```python
from build123d import *

# Parameters (mm, degrees)
F0_W     = 67
F0_H     = 88
F1_DEPTH = 3
F2_R     = 3.9
F3_DEPTH = 3.81
F5_D     = 3.5


with BuildPart() as f1:
    # F0 (on Top) → F1 (new body)
    with BuildSketch(Plane.XY):
        Rectangle(F0_W, F0_H)
    extrude(amount=F1_DEPTH)

    # F2 (on face) → F3 (join)
    with BuildSketch(Plane.XY.offset(3)):
        with Locations((-29.5, 40)):
            Circle(F2_R)
        with Locations((29.5, 40)):
            Circle(F2_R)
        with Locations((-29.5, -40)):
            Circle(F2_R)
        with Locations((29.5, -40)):
            Circle(F2_R)
    extrude(amount=F3_DEPTH)

    # F5 (through all)
    with Locations(Plane(origin=(0, 0, 0), x_dir=(1, 0, 0), z_dir=(0, 0, -1))):
        with Locations((29.5, 40), (-29.5, 40), (-29.5, -40), (29.5, -40)):
            Hole(F5_D / 2)


solid = f1.part
```
Input: part model. Units: mm. Frame: model coordinates. A direction names the side the tool comes from. Round coordinates to 2 decimals unless told otherwise and drop trailing zeros. Loops run counter-clockwise (first coordinate to the right, second up) from the corner with the lowest first, then second, coordinate; pieces in that order, holes last.
1) Section query D-D on x = 0.5. Return the cut outline in (y, z).
Ans:
outline: (-44, 0) - (44, 0) - (44, 3) - (-44, 3) - close
2) Pull-direction query (X, two-part tool) for faces 3 (the flat face through (0, 44, 1)), 4 (the flat face through (33.5, -1, 1)), 5 (the cylindrical face through (26.405, -42.373, 4.878)); classes: released by +X, released by -X, zero draft, split by the parting line, or undercut.
Ans:
face 3: zero draft
face 4: released by +X
face 5: undercut
3) Material intervals for line 1 (Y direction, x = 29.5, z = 3.5); line 2 (X direction, y = 40, z = 2.5); line 3 (Y direction, x = 29.5, z = 2.5), sorted ascending.
Ans:
line 1: y = -43.9 to -41.75, -38.25 to -36.1, 36.1 to 38.25, 41.75 to 43.9
line 2: x = -33.5 to -31.25, -27.75 to 27.75, 31.25 to 33.5
line 3: y = -44 to -41.75, -38.25 to 38.25, 41.75 to 44
4) Section query B-B on x = 29.5. Return the cut outline in (y, z), plus the area to 3 significant figures.
Ans:
outline: (-44, 0) - (-41.75, 0) - (-41.75, 6.81) - (-43.9, 6.81) - (-43.9, 3) - (-44, 3) - close; (-38.25, 0) - (38.25, 0) - (38.25, 6.81) - (36.1, 6.81) - (36.1, 3) - (-36.1, 3) - (-36.1, 6.81) - (-38.25, 6.81) - close; (41.75, 0) - (44, 0) - (44, 3) - (43.9, 3) - (43.9, 6.81) - (41.75, 6.81) - close
area: 276 mm2
5) Set-up query: faces 1 (the cylindrical face through (-32.595, -42.373, 4.878)), 2 (the flat face through (-29, 38, 6.81)). Return all of +Z, -Z, +X, -X, +Y, -Y with unobstructed straight access to the full face (end or side cutting, diameter ignored); none if empty.
Ans:
face 1: +Z
face 2: +Z, +X, -X, +Y, -Y
6) Section query C-C on y = -40. Return the cut outline in (x, z).
Ans:
outline: (-33.5, 0) - (-31.25, 0) - (-31.25, 6.81) - (-33.4, 6.81) - (-33.4, 3) - (-33.5, 3) - close; (-27.75, 0) - (27.75, 0) - (27.75, 6.81) - (25.6, 6.81) - (25.6, 3) - (-25.6, 3) - (-25.6, 6.81) - (-27.75, 6.81) - close; (31.25, 0) - (33.5, 0) - (33.5, 3) - (33.4, 3) - (33.4, 6.81) - (31.25, 6.81) - close
7) Section query A-A on z = 5.5. Return the cut outline in (x, y).
Ans:
outline: circle Ø7.8 at (-29.5, -40); circle Ø7.8 at (-29.5, 40); circle Ø7.8 at (29.5, -40); circle Ø7.8 at (29.5, 40); hole circle Ø3.5 at (-29.5, -40); hole circle Ø3.5 at (-29.5, 40); hole circle Ø3.5 at (29.5, -40); hole circle Ø3.5 at (29.5, 40)
8) Pin query (flat end, axial travel): pin 1 (3 mm diameter, centred on x = -23.5, y = 22.5, fed in from +Z); pin 2 (1.5 mm diameter, centred on y = 18, z = 4, fed in from +X). Return the tip coordinate at first contact, or that it passes through.
Ans:
pin 1: stops at z = 3
pin 2: passes through
